Answer from the drawing. Dimensions are ordinates in mm from the lowest x, y and z of the part. A direction names the side the tool comes from. Give positions to 0.01 mm unless a question says otherwise; leave off trailing zeros. Write each loop counter-clockwise with the first axis right and the second up, starting at its lowest first coordinate (ties: lowest second). Pieces come first, ordered by that corner, then holes.
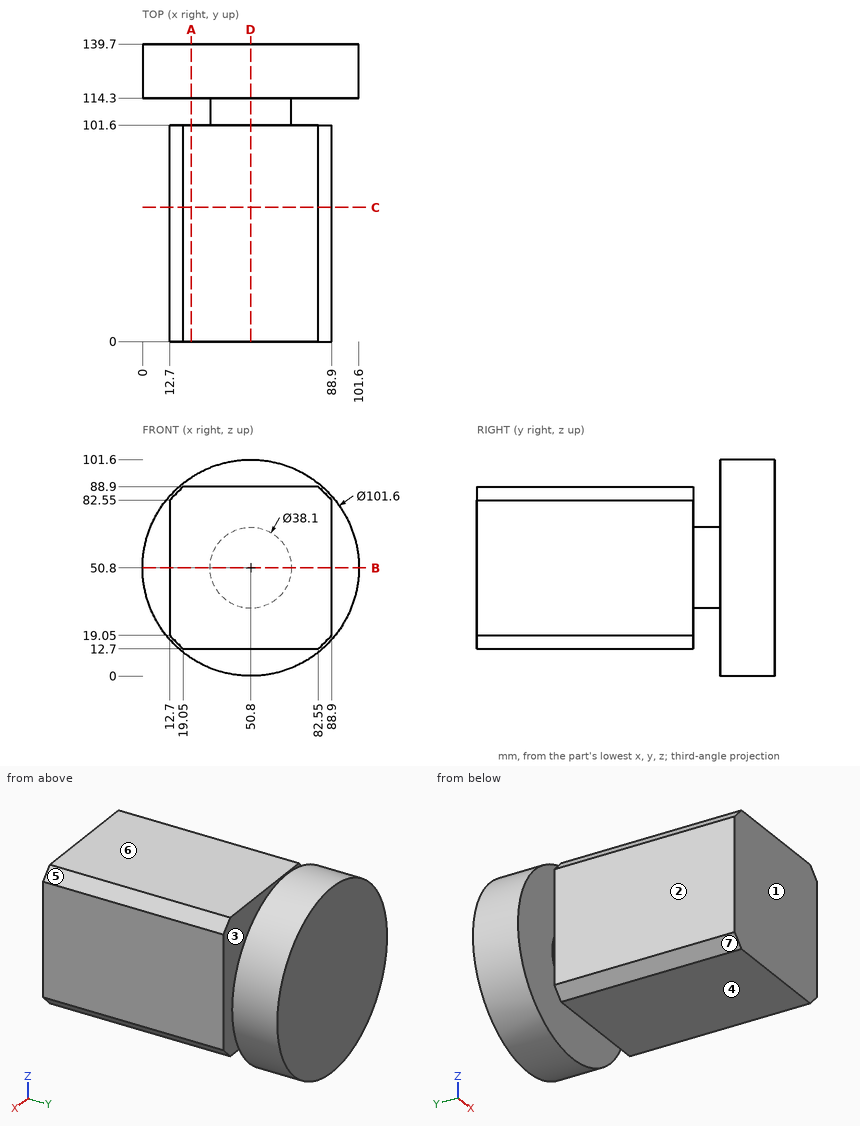
Item 1: Section A-A (x = 23) is taken. Write down the section's boundary in (y, z).
Result set:
outline: (0, 12.7) - (101.6, 12.7) - (101.6, 88.9) - (0, 88.9) - close; (114.3, 8.28) - (139.7, 8.28) - (139.7, 93.32) - (114.3, 93.32) - close
Item 2: Section B-B (z = 50.8) is taken. Write down the section's boundary in (x, y), and give its area (3 significant figures).
Result set:
outline: (0, 114.3) - (31.75, 114.3) - (31.75, 101.6) - (12.7, 101.6) - (12.7, 0) - (88.9, 0) - (88.9, 101.6) - (69.85, 101.6) - (69.85, 114.3) - (101.6, 114.3) - (101.6, 139.7) - (0, 139.7) - close
area: 10,800 mm2
Item 3: Determine the mould class of the marked faces 1, 2 and 3 for opening direction Y: pulls with the +Y half, pulls with the -Y half, needs draft (parallel to the pull), parting line crosses it, or undercut.
Result set:
face 1: pulls with the -Y half
face 2: needs draft
face 3: undercut
Item 4: Section D-D (x = 50.8) is taken. Write down the section's boundary in (y, z).
Result set:
outline: (0, 12.7) - (101.6, 12.7) - (101.6, 31.75) - (114.3, 31.75) - (114.3, 0) - (139.7, 0) - (139.7, 101.6) - (114.3, 101.6) - (114.3, 69.85) - (101.6, 69.85) - (101.6, 88.9) - (0, 88.9) - close
Item 5: Which of the six approach directions +Z, -Z, +X, -X, +Y, -Y give full straight-line access (tool end or side, diameter ignored) to the marked faces 4, 5, 6 and 7?
Result set:
face 4: -Z, +X, -X, -Y
face 5: +Z, +X, -Y
face 6: +Z, +X, -X, -Y
face 7: -Z, -X, -Y
Item 6: Section C-C (y = 63) is taken. Write down the section's boundary in (x, z).
Result set:
outline: (12.7, 19.05) - (19.05, 12.7) - (82.55, 12.7) - (88.9, 19.05) - (88.9, 82.55) - (82.55, 88.9) - (19.05, 88.9) - (12.7, 82.55) - close
Item 7: Each of these flat-tipped pins is pushed along its axis until it touches: pin 1 Ø8 at (x, z) = (41.5, 68) entering from -Y; pin 2 Ø5 at (y, z) = (43.5, 59.5) entering from +X; pin 3 Ø5 at (y, z) = (46, 47) entering from -X; pin 4 Ø6 at (x, y) = (51.5, 121.5) entering from -Z. Where does it stop, or does it pass through?
Result set:
pin 1: stops at y = 0
pin 2: stops at x = 88.9
pin 3: stops at x = 12.7
pin 4: stops at z = 0
Item 8: Find the intervals of material crossed by line 1 along Y through (x, z) = (71.5, 76); line 2 along Y through (x, z) = (52, 92.5); line 3 along X through (y, z) = (26.5, 36), in increasing order.
Result set:
line 1: y = 0 to 101.6, 114.3 to 139.7
line 2: y = 114.3 to 139.7
line 3: x = 12.7 to 88.9
